Read the model definition and answer for the solid it produces. Units are mm, in the model's axes. Round coordinates to 2 decimals unless told otherwise and drop trailing zeros. Write each loop counter-clockwise with the first axis right and the second up, starting at its lowest first coordinate (ties: lowest second). Pieces come first, ordered by that corner, then holes.
from build123d import *

# Parameters (mm, degrees)
F0_R     = 3
F1_DEPTH = 4
F2_R     = 5


# Not quite as in the source:
# - a fillet or chamfer that OpenCascade refuses, or shapes differently, is made with other operations: its cross-section is extruded or revolved along the edge and cut away or added


with BuildPart() as f1:
    # F0 (on Front) → F1 (new body)
    with BuildSketch(Plane.XZ):
        Polygon((45.8173750394, -79.3580214376), (45.8173750394, 79.3580214376), (-91.6347500787, 0), align=None)
        with Locations((30.8173750394, -53.3772593241)):
            Circle(F0_R, mode=Mode.SUBTRACT)
        with Locations((-61.6347500787, 0)):
            Circle(F0_R, mode=Mode.SUBTRACT)
        Circle(F0_R, mode=Mode.SUBTRACT)
        with Locations((30.8173750394, 53.3772593241)):
            Circle(F0_R, mode=Mode.SUBTRACT)
    extrude(amount=F1_DEPTH)

    # F2
    f2_edges = [f1.edges().sort_by_distance(p)[0] for p in [
        (45.817375, -2, 79.358021),
        (45.817375, -2, -79.358021),
        (-91.63475, -2, 0),
    ]]
    fillet(f2_edges, radius=F2_R)

    # F3: chamfer of 5 on 4 edges, made by hand

    # F3_s1 → F3_t2 (revolve, cut)
    with BuildSketch(Plane.XY):
        Polygon((8, 0), (3, -5), (3, 0), align=None)
    revolve(axis=Axis((0, 0, 0), (0, -1, 0)), mode=Mode.SUBTRACT)

    # F3_s3 → F3_t4 (revolve, cut)
    with BuildSketch(Plane.XY):
        Polygon((-53.6347500787, -4), (-58.6347500787, 1), (-58.6347500787, -4), align=None)
    revolve(axis=Axis((-61.6347500787, -4, 0), (0, -1, 0)), mode=Mode.SUBTRACT)

    # F3_s5 → F3_t6 (revolve, cut)
    with BuildSketch(Plane.XY.offset(53.3772593241)):
        Polygon((38.8173750394, -4), (33.8173750394, 1), (33.8173750394, -4), align=None)
    revolve(axis=Axis((30.8173750394, -4, 53.3772593241), (0, -1, 0)), mode=Mode.SUBTRACT)

    # F3_s7 → F3_t8 (revolve, cut)
    with BuildSketch(Plane.XY.offset(-53.3772593241)):
        Polygon((38.8173750394, -4), (33.8173750394, 1), (33.8173750394, -4), align=None)
    revolve(axis=Axis((30.8173750394, -4, -53.3772593241), (0, -1, 0)), mode=Mode.SUBTRACT)


solid = f1.part
Q1. Section B-B (y = -1) is taken. Determine the outline of the cut face in (x, z), then the cut area to 3 significant figures.
Verdict:
outline: (-84.13, -4.33) - (38.32, -75.03) arc R5 ccw to (45.82, -70.7) - (45.82, 70.7) arc R5 ccw to (38.32, 75.03) - (-84.13, 4.33) arc R5 ccw to start; hole circle Ø10 at (-61.63, 0); hole circle Ø14 at (0, 0); hole circle Ø10 at (30.82, -53.38); hole circle Ø10 at (30.82, 53.38)
area: 10,500 mm2
Q2. Section D-D (z = -31.5) is taken. Determine the outline of the cut face in (x, y), then the cut area to 3 significant figures.
Verdict:
outline: (-37.08, -4) - (45.82, -4) - (45.82, 0) - (-37.08, 0) - close
area: 332 mm2
Q3. Section A-A (x = 0) is taken. Determine the outline of the cut face in (y, z).
Verdict:
outline: (-4, -52.91) - (0, -52.91) - (0, -8) - (-4, -4) - close; (-4, 4) - (0, 8) - (0, 52.91) - (-4, 52.91) - close
Q4. Determine the mould class of faces 1 (the conical face through (-64.96, -0.19, -2.55)), 2 (the flat face through (-7, -4, 1)), 3 (the flat face through (-22.052, -1.972, 40.174)), 4 (the cylindrical face through (43.38, -2.03, 74.99)) for opening direction X: pulls with the +X half, pulls with the -X half, needs draft (parallel to the pull), parting line crosses it, or undercut.
Verdict:
face 1: undercut
face 2: needs draft
face 3: pulls with the -X half
face 4: parting line crosses it
Q5. Straight lines are drawn through the part: probe 1 along Z at (x, y) = (27, -3.2); probe 2 along Z at (x, y) = (31.5, -0.85); probe 3 along X at (y, z) = (-1.45, 56). For each, find the intervals that lie inside material, in ascending order.
Verdict:
probe 1: z = -68.49 to -59.48, -47.27 to 47.27, 59.48 to 68.49
probe 2: z = -71.09 to -58.18, -48.58 to 48.58, 58.18 to 71.09
probe 3: x = 5.36 to 26.04, 35.59 to 45.82
Q6. Section C-C (z = 0) is taken. Determine the outline of the cut face in (x, y).
Verdict:
outline: (-86.63, -4) - (-69.63, -4) - (-65.63, 0) - (-86.63, 0) - close; (-57.63, 0) - (-53.63, -4) - (-4, -4) - (-8, 0) - close; (4, -4) - (45.82, -4) - (45.82, 0) - (8, 0) - close
